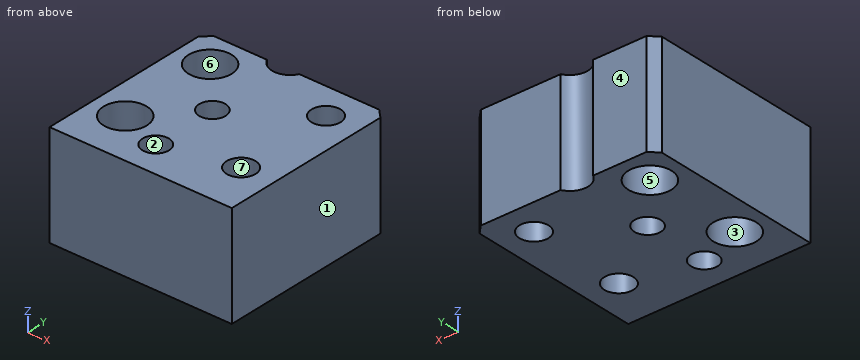
```python
from build123d import *

# Parameters (mm, degrees)
SKIZZE1_W                                            = 110
SKIZZE1_H                                            = 62.3
AUFSATZ_LINEAR_AUSTRAGEN1_DEPTH                      = 110
DURCHGANGSLOCH_F_R_M161_D                            = 17.5
STIRNSENKUNG_F_R_M16_ZYLINDERSCHRAUBE_MI_D           = 17.5
STIRNSENKUNG_F_R_M16_ZYLINDERSCHRAUBE_MI_CBORE_D     = 26
STIRNSENKUNG_F_R_M16_ZYLINDERSCHRAUBE_MI_CBORE_DEPTH = 16.6
F_16_0_H7_16_DURCHMESSER_BOHRUNG2_D                  = 16
F_22_0_22_DURCHMESSER_BOHRUNG1_D                     = 22
FASE1_SIZE                                           = 5
STIRNSENKUNG_F_R_M16_ZYLINDERSCHRAUB_2_D             = 17.5
STIRNSENKUNG_F_R_M16_ZYLINDERSCHRAUB_2_CBORE_D       = 26
STIRNSENKUNG_F_R_M16_ZYLINDERSCHRAUB_2_CBORE_DEPTH   = 16.6


with BuildPart() as part:
    # Skizze1 → Aufsatz-Linear austragen1 (new body)
    with BuildSketch(Plane(origin=(0, 0, 0), x_dir=(1, 0, 0), z_dir=(0, 1, 0))):
        Rectangle(SKIZZE1_W, SKIZZE1_H)
    extrude(amount=AUFSATZ_LINEAR_AUSTRAGEN1_DEPTH)

    # Durchgangsloch für M161 (through all)
    with Locations(Plane.XY.offset(31.15)):
        with Locations((35, 90), (35, 30)):
            Hole(DURCHGANGSLOCH_F_R_M161_D / 2)

    # Stirnsenkung f_r M16 Zylinderschraube mi (through all)
    with Locations(Plane.XY.offset(31.15)):
        with Locations((-35, 90), (-35, 30)):
            CounterBoreHole(STIRNSENKUNG_F_R_M16_ZYLINDERSCHRAUBE_MI_D / 2, STIRNSENKUNG_F_R_M16_ZYLINDERSCHRAUBE_MI_CBORE_D / 2, STIRNSENKUNG_F_R_M16_ZYLINDERSCHRAUBE_MI_CBORE_DEPTH)

    # Ø16.0 H7 (16) Durchmesser Bohrung2 (through all)
    with Locations(Plane(origin=(0, 0, -31.15), x_dir=(-1, 0, 0), z_dir=(0, 0, -1))):
        with Locations((8, 60), (8, 20)):
            Hole(F_16_0_H7_16_DURCHMESSER_BOHRUNG2_D / 2)

    # Ø22.0 (22) Durchmesser Bohrung1 (through all)
    with Locations(Plane(origin=(0, 0, -31.15), x_dir=(-1, 0, 0), z_dir=(0, 0, -1))):
        with Locations((8, 115)):
            Hole(F_22_0_22_DURCHMESSER_BOHRUNG1_D / 2)

    # Fase1
    fase1_edges = [part.edges().sort_by_distance(p)[0] for p in [
        (-55, 110, 0),
        (55, 110, 0),
    ]]
    chamfer(fase1_edges, length=FASE1_SIZE)

    # Stirnsenkung f_r M16 Zylinderschraub 2 (through all)
    with Locations(Plane(origin=(0, 0, -31.15), x_dir=(-1, 0, 0), z_dir=(0, 0, -1))):
        with Locations((35, 90), (35, 30)):
            CounterBoreHole(STIRNSENKUNG_F_R_M16_ZYLINDERSCHRAUB_2_D / 2, STIRNSENKUNG_F_R_M16_ZYLINDERSCHRAUB_2_CBORE_D / 2, STIRNSENKUNG_F_R_M16_ZYLINDERSCHRAUB_2_CBORE_DEPTH)


solid = part.part
```
Here's how the part is built. I have some questions about the finished solid (model axes, mm). Face numbers are marked on the shaded views. A direction names the side the tool comes from. Coordinates: 2 decimals unless noted, no trailing zeros. Order: outer loops, then holes, each group sorted by start corner. A loop starts at its lowest first (then second) coordinate and runs counter-clockwise, first axis right, second up.
1) Which directions (+Z, -Z, +X, -X, +Y, -Y) give clear straight access to the entire face, cutting with the end or side of a thin tool? Please do the marked faces 5, 6 and 7.
2) Imagine slicing it at A-A on x = 35. List the corners of the cut face in (y, z) for me, and give its area (3 significant figures).
3) I need wall thicknesses on line 1 (Y direction, x = -35, z = 22); line 2 (Y direction, x = -37, z = -10.5); line 3 (X direction, y = 31, z = 13.5). Which ranges of each line are inside material? Lowest first, please.
4) Imagine slicing it at D-D on y = 60. List the corners of the cut face in (x, z) for me, and give its area (3 significant figures).
5) We'd pull the mould along Y, two halves only. Please class the marked faces 1, 2, 3 and 4: +Y half, -Y half, draft (parallel to the pull), parting line (faces both ways), or undercut.
6) Imagine slicing it at B-B on z = 22. List the corners of the cut face in (x, y) for me.
7) Imagine slicing it at C-C on y = 30. List the corners of the cut face in (x, z) for me, and give its area (3 significant figures).
8) Will these pins go through, and if not, where does the flat tip stop? pin 1 (23.5 mm diameter, centred on x = -35, y = 90, fed in from +Z); pin 2 (15.5 mm diameter, centred on x = -35, y = 30, fed in from -Z); pin 3 (13 mm diameter, centred on x = -39, y = 86, fed in from -Z).
Response values:
1. face 5: -Z
1. face 6: +Z
1. face 7: +Z, -Z
2. outline: (0, -31.15) - (21.25, -31.15) - (21.25, 31.15) - (0, 31.15) - close; (38.75, -31.15) - (81.25, -31.15) - (81.25, 31.15) - (38.75, 31.15) - close; (98.75, -31.15) - (110, -31.15) - (110, 31.15) - (98.75, 31.15) - close
2. area: 4,670 mm2
3. line 1: y = 0 to 17, 43 to 77, 103 to 110
3. line 2: y = 0 to 21.48, 38.52 to 81.48, 98.52 to 110
3. line 3: x = -55 to -43.69, -26.31 to 26.31, 43.69 to 55
4. outline: (-55, -31.15) - (-16, -31.15) - (-16, 31.15) - (-55, 31.15) - close; (0, -31.15) - (55, -31.15) - (55, 31.15) - (0, 31.15) - close
4. area: 5,860 mm2
5. face 1: draft
5. face 2: undercut
5. face 3: undercut
5. face 4: +Y half
6. outline: (-55, 0) - (55, 0) - (55, 105) - (50, 110) - (1.8, 110) arc R11 cw to (-17.8, 110) - (-50, 110) - (-55, 105) - close; hole circle Ø26 at (-35, 30); hole circle Ø26 at (-35, 90); hole circle Ø16 at (-8, 20); hole circle Ø16 at (-8, 60); hole circle Ø17.5 at (35, 30); hole circle Ø17.5 at (35, 90)
7. outline: (-55, -31.15) - (-48, -31.15) - (-48, -14.55) - (-43.75, -14.55) - (-43.75, 14.55) - (-48, 14.55) - (-48, 31.15) - (-55, 31.15) - close; (-26.25, -14.55) - (-22, -14.55) - (-22, -31.15) - (26.25, -31.15) - (26.25, 31.15) - (-22, 31.15) - (-22, 14.55) - (-26.25, 14.55) - close; (43.75, -31.15) - (55, -31.15) - (55, 31.15) - (43.75, 31.15) - close
7. area: 4,390 mm2
8. pin 1: stops at z = 14.55
8. pin 2: passes through
8. pin 3: stops at z = -14.55
